Could you check a few things on this drawing? It's one solid part, dimensions in mm from its lowest x, y, z. A direction names the side the tool comes from. Give positions to 0.01 mm unless a question says otherwise; leave off trailing zeros. Loops run counter-clockwise (first coordinate to the right, second up) from the corner with the lowest first, then second, coordinate; pieces in that order, holes last. Notation, with made-up numbers: M 39,11 L 70,11 A16 ccw 70,34 Z; hole C -25.5,-34 d2. An arc over 180 degrees is marked long. Answer as a JSON object with one key per item and string values.
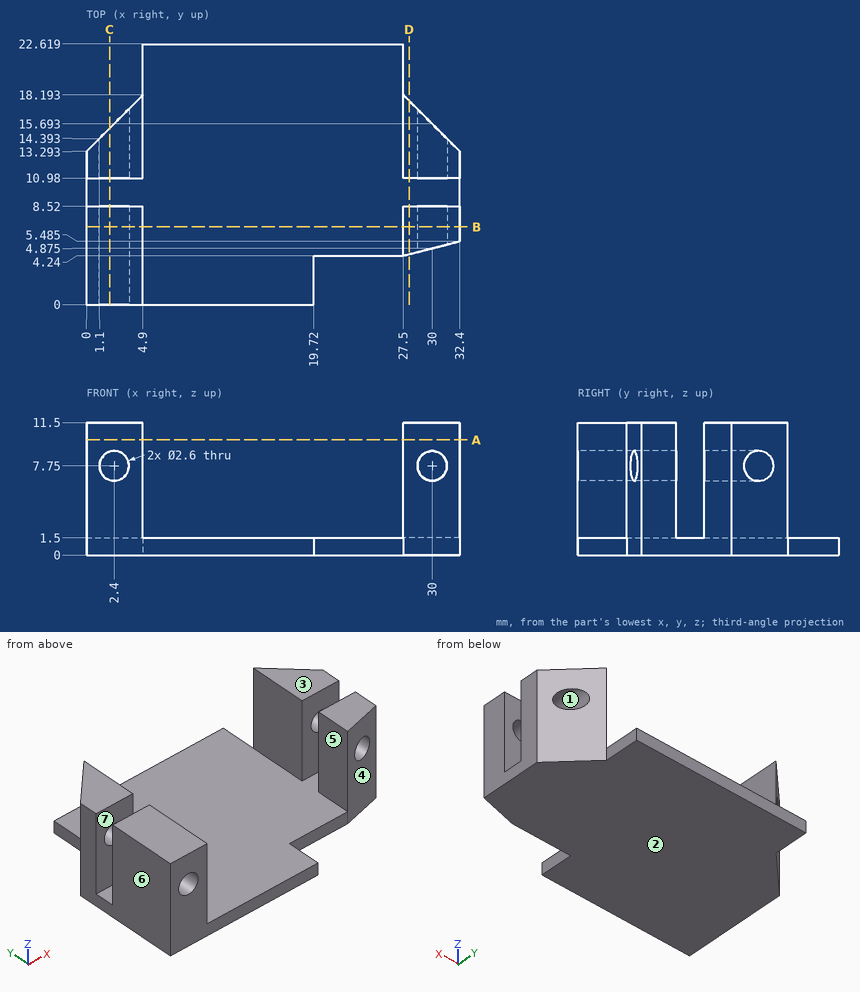
1) If we mould it in two halves opening along Z, with no side actions, what happens to the marked faces 1, 2, 3 and 4? For each: +Z half, -Z half, draft (parallel to the pull), parting line (faces both ways), or undercut.
Answer list:
{"face 1": "undercut", "face 2": "-Z half", "face 3": "+Z half", "face 4": "draft"}
2) Suppose I cut it at B-B, the plane y = 6.75. Write out the boundary of the cut face in (x, z), and give its area (3 significant figures).
Answer list:
{"outline": "M 0,0 L 32.4,0 L 32.4,11.5 L 27.5,11.5 L 27.5,1.5 L 4.9,1.5 L 4.9,11.5 L 0,11.5 Z; hole C 2.4,7.75 d2.6; hole C 30,7.75 d2.6", "area": "136 mm^2"}
3) Suppose I cut it at A-A, the plane z = 10. Write out the boundary of the cut face in (x, y) (1 decimal), and give its area (3 significant figures).
Answer list:
{"outline": "M 0,0 L 4.9,0 L 4.9,8.5 L 0,8.5 Z; M 0,11 L 4.9,11 L 4.9,18.2 L 0,13.3 Z; M 27.5,4.2 L 32.4,5.5 L 32.4,8.5 L 27.5,8.5 Z; M 27.5,11 L 32.4,11 L 32.4,13.3 L 27.5,18.2 Z", "area": "106 mm^2"}
4) For the marked faces 5, 6 and 7, which set-ups out of +Z, -Z, +X, -X, +Y, -Y let a thin tool reach every point of the face, with its end or its side?
Answer list:
{"face 5": "+Z, +Y, -Y", "face 6": "+Z, -Z, -X, +Y, -Y", "face 7": "+Z, +X, -X"}
5) Please list where these lines run through material, in increasing order: line 1 along X through (y, z) = (7.1, 7.75); line 2 along X through (y, z) = (5, 7.75); line 3 along X through (y, z) = (11.75, 3.5). Write a range as from..to.
Answer list:
{"line 1": "0..1.1, 3.7..4.9, 27.5..28.7, 31.3..32.4", "line 2": "0..1.1, 3.7..4.9, 27.5..28.7", "line 3": "0..4.9, 27.5..32.4"}
6) Will these pins go through, and if not, where does the flat tip stop? pin 1 Ø1.5 at (x, z) = (1.5, 6) entering from -Y; pin 2 Ø8 at (x, y) = (22, 14.5) entering from +Z; pin 3 Ø1.6 at (x, z) = (30, 7.75) entering from -Y; pin 4 Ø1.2 at (y, z) = (20.5, 0.5) entering from -X.
Answer list:
{"pin 1": "y = 0", "pin 2": "z = 1.5", "pin 3": "through", "pin 4": "x = 4.9"}
7) Suppose I cut it at D-D, the plane x = 28. Write out the boundary of the cut face in (y, z), and give its area (3 significant figures).
Answer list:
{"outline": "M 4.37,0 L 17.69,0 L 17.69,11.5 L 10.98,11.5 L 10.98,1.5 L 8.52,1.5 L 8.52,11.5 L 4.37,11.5 Z", "area": "129 mm^2"}
8) Suppose I cut it at C-C, the plane x = 2. Write out the boundary of the cut face in (y, z).
Answer list:
{"outline": "M 0,0 L 15.29,0 L 15.29,6.51 L 10.98,6.51 L 10.98,1.5 L 8.52,1.5 L 8.52,6.51 L 0,6.51 Z; M 0,8.99 L 8.52,8.99 L 8.52,11.5 L 0,11.5 Z; M 10.98,8.99 L 15.29,8.99 L 15.29,11.5 L 10.98,11.5 Z"}
